```python
from build123d import *

# Parameters (mm, degrees)
F0_R     = 12.7
F1_DEPTH = 60.325
F3_W     = 32.8422
F3_H     = 41.275
F6_DEPTH = 34.798
F7_DEPTH = 19.05
F5_W     = 50.4518977821
F5_H     = 22.3266
F5_R     = 6.35
F8_DEPTH = 47.498
F9_R     = 3.302


with BuildPart() as f1:
    # F0 (on Front) → F1 (new body)
    with BuildSketch(Plane.XZ):
        with BuildLine():
            ThreePointArc((-79.7361564685, 22.352), (-117.8934072416, 38.1572507731), (-102.0881564685, 0))
            Line((-102.0881564685, 0), (92.1202435315, 0))
            Line((92.1202435315, 0), (92.1202435315, 14.478))
            ThreePointArc((92.1202435315, 14.478), (89.8140023266, 20.0457587951), (84.2462435315, 22.352))
            Line((84.2462435315, 22.352), (48.0004435315, 22.352))
            Line((48.0004435315, 22.352), (48.0004435315, 52.07))
            ThreePointArc((48.0004435315, 52.07), (46.5125459799, 55.6621024484), (42.9204435315, 57.15))
            Line((42.9204435315, 57.15), (28.9504435315, 57.15))
            ThreePointArc((28.9504435315, 57.15), (25.3762588931, 38.4343576341), (15.1582435315, 22.352))
            Line((15.1582435315, 22.352), (-79.7361564685, 22.352))
        make_face()
        with Locations((-102.0881564685, 22.352)):
            Circle(F0_R, mode=Mode.SUBTRACT)
    extrude(amount=-F1_DEPTH)

    # F3 (on offset) → F6 (cut, through all)
    with BuildSketch(Plane.XY.offset(22.352)):
        with Locations((31.5793435315, 39.6875)):
            Rectangle(F3_W, F3_H)
    extrude(amount=F6_DEPTH, mode=Mode.SUBTRACT)

    # F4 (on Front) → F7 (cut)
    with BuildSketch(Plane.XZ):
        Polygon((15.1582435315, 0), (15.1582435315, 22.352), (-16.2361564685, 22.352), (-10.2417564685, 0), align=None)
    extrude(amount=-F7_DEPTH, mode=Mode.SUBTRACT)

    # F5 (on offset) → F8 (cut, symmetric)
    with BuildSketch(Plane.XY.offset(22.352)):
        with Locations((-104.9621053595, 30.1625)):
            Rectangle(F5_W, F5_H)
        with Locations((53.2582435315, 37.973)):
            Circle(F5_R)
    extrude(amount=F8_DEPTH, both=True, mode=Mode.SUBTRACT)

    # F9
    f9_edges = [f1.edges().sort_by_distance(p)[0] for p in [
        (-79.736156, 9.4996, 22.352),
        (-79.736156, 50.8254, 22.352),
    ]]
    fillet(f9_edges, radius=F9_R)


solid = f1.part
```
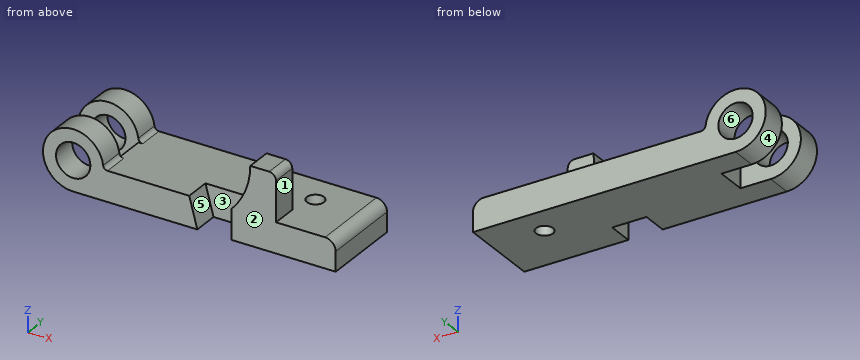
Can you work these out from the model? Positions are in its coordinate system, mm. Face numbers are marked on the shaded views. A direction names the side the tool comes from. Coordinates: 2 decimals unless noted, no trailing zeros. Loops run counter-clockwise (first coordinate to the right, second up) from the corner with the lowest first, then second, coordinate; pieces in that order, holes last. Notation, with made-up numbers: (9.25, 73.5) -> (30.25, 73.5) arc R18 cw to (30.25, 81.5) -> close; hole circle Ø11 at (10, 36.25). An arc over 180 degrees is marked (long way). Put each result on its own line as item: value. Start each with the question number.
Q1. If I drill on line 1 (Y direction, x = -93.5, z = 12) (3 decimals); line 2 (Z direction, x = -102, y = 47.5); line 3 (X direction, y = 17.5, z = 18.5), over which ranges is the centre line in solid material (lowest first)? Write a range as [from, to].
Q2. I want a section at A-A (y = 14.5). Write out the boundary of the cut face in (x, z), plus the area to 3 significant figures.
Q3. I want a section at C-C (y = 47.5). Write out the boundary of the cut face in (x, z).
Q4. I'm going to push flat-ended pins straight in: P1, Ø18, axis at y = 27.5, z = 14.5, coming from the -X side; P2, Ø15, axis at x = -102.09, z = 22.35, coming from the -Y side; P3, Ø3, axis at x = -86, y = 14, coming from the +Z side; P4, Ø1, axis at x = -73, y = 37, coming from the +Z side. Where does each tip first touch, or does it pass through?
Q5. For the marked faces 5 and 6, which set-ups out of +Z, -Z, +X, -X, +Y, -Y let a thin tool reach every point of the face, with its end or its side?
Q6. I want a section at B-B (x = 50.5). Write out the boundary of the cut face in (y, z) (3 decimals).
Q7. I want a section at D-D (x = -50). Write out the boundary of the cut face in (y, z) (3 decimals), plus the area to 3 significant figures.
Q8. Thinking about a two-plate mould opening in X: for the marked faces 1, 2, 3 and 4, which applies, pulls with the +X half, pulls with the -X half, needs draft (parallel to the pull), parting line crosses it, or undercut?
Taken from the geometry:
1. line 1: y = [0, 18.999], [41.326, 60.325]
1. line 2: z = [0, 9.65], [35.05, 44.7]
1. line 3: x = [-124.11, -114.19], [-89.99, -15.2], [15.16, 91.02]
2. outline: (-102.09, 0) -> (-10.24, 0) -> (-16.24, 22.35) -> (-76.65, 22.35) arc R3.3 cw to (-79.92, 25.23) arc R22.35 ccw (long way) to start; (15.16, 0) -> (92.12, 0) -> (92.12, 14.48) arc R7.87 ccw to (84.25, 22.35) -> (48, 22.35) -> (48, 52.07) arc R5.08 ccw to (42.92, 57.15) -> (28.95, 57.15) arc R50.8 cw to (15.16, 22.35) -> close; hole circle Ø25.4 at (-102.09, 22.35)
2. area: 5,170 mm2
3. outline: (-102.09, 0) -> (92.12, 0) -> (92.12, 14.48) arc R7.87 ccw to (84.25, 22.35) -> (-76.65, 22.35) arc R3.3 cw to (-79.92, 25.23) arc R22.35 ccw (long way) to start; hole circle Ø25.4 at (-102.09, 22.35)
4. P1: stops at x = -123.9
4. P2: passes through
4. P3: stops at z = 39.29
4. P4: stops at z = 22.35
5. face 5: +Z, -Y
5. face 6: +Y, -Y
6. outline: (0, 0) -> (32.253, 0) -> (32.253, 22.352) -> (0, 22.352) -> close; (43.693, 0) -> (60.325, 0) -> (60.325, 22.352) -> (43.693, 22.352) -> close
7. outline: (0, 0) -> (60.325, 0) -> (60.325, 22.352) -> (0, 22.352) -> close
7. area: 1,350 mm2
8. face 1: pulls with the +X half
8. face 2: needs draft
8. face 3: undercut
8. face 4: parting line crosses it
